Part model, mm, in its own coordinate system. Round coordinates to 2 decimals unless told otherwise and drop trailing zeros. Loops run counter-clockwise (first coordinate to the right, second up) from the corner with the lowest first, then second, coordinate; pieces in that order, holes last. Notation, with made-up numbers: M 37.25,-10.5 L 55.25,-10.5 A28 cw 55.25,8.5 Z; hole C -4.75,-39 d9. An arc over 180 degrees is marked long. Put each result on its own line as item: value. Start each with the question number.
1) Slice it at A-A on x = -97. Give the cut face in (y, z), then the cut area to 3 significant figures.
2) Probe line 1 along X through (y, z) = (2.75, -69); line 2 along X through (y, z) = (2, -39.5); line 3 along X through (y, z) = (5, 8). List the from-to ranges inside material, lowest first.
3) Slice it at B-B on y = 5. State how many separate pieces and enclosed holes the cut face has, then the cut area to 3 significant figures.
4) Drop a flat-ended pin along its axis: pin 1 Ø2 at (x, z) = (-12, 25) entering from +Y. Give the stop position or say it passes through.
```python
from build123d import *

# Parameters (mm, degrees)
SKETCH_1_R      = 1.7
SKETCH_1_R_2    = 2.15
SKETCH_1_R_3    = 2.65
SKETCH_1_R_4    = 10
EXTRUDE_2_DEPTH = 6


with BuildPart() as part:
    # 草图1 → 凸台-拉伸2 (new body)
    with BuildSketch(Plane(origin=(0, 0, 0), x_dir=(1, 0, 0), z_dir=(0, 1, 0))):
        with BuildLine():
            ThreePointArc((-125, -42), (-122.071067812, -49.071067812), (-115, -52))
            Line((-115, -52), (115, -52))
            ThreePointArc((115, -52), (122.071067812, -49.071067812), (125, -42))
            Line((125, -42), (125, 129))
            ThreePointArc((125, 129), (122.071067812, 136.071067812), (115, 139))
            Line((115, 139), (54.15581278, 139))
            ThreePointArc((54.15581278, 139), (50.06955504, 138.127020198), (46.696741396, 135.660499537))
            ThreePointArc((46.696741396, 135.660499537), (38.879992551, 123.497665763), (35.221472878, 109.510124102))
            ThreePointArc((35.221472878, 109.510124102), (33.603401462, 106.295315162), (30.245528585, 105))
            Line((30.245528585, 105), (-30.245528585, 105))
            ThreePointArc((-30.245528585, 105), (-33.603401462, 106.295315162), (-35.221472878, 109.510124102))
            ThreePointArc((-35.221472878, 109.510124102), (-38.879992551, 123.497665763), (-46.696741396, 135.660499537))
            ThreePointArc((-46.696741396, 135.660499537), (-50.06955504, 138.127020198), (-54.15581278, 139))
            Line((-54.15581278, 139), (-115, 139))
            ThreePointArc((-115, 139), (-122.071067812, 136.071067812), (-125, 129))
            Line((-125, 129), (-125, -42))
        make_face()
        with Locations(Location((-120, -35, 0), (0, 0, 270))):
            Circle(SKETCH_1_R, mode=Mode.SUBTRACT)
        with Locations(Location((-52, -35, 0), (0, 0, 270))):
            Circle(SKETCH_1_R, mode=Mode.SUBTRACT)
        with Locations(Location((-35, -25, 0), (0, 0, 270))):
            Circle(SKETCH_1_R_2, mode=Mode.SUBTRACT)
        with Locations(Location((-24.5, -25, 0), (0, 0, 270))):
            Circle(SKETCH_1_R, mode=Mode.SUBTRACT)
        with Locations(Location((-12, -25, 0), (0, 0, 270))):
            Circle(SKETCH_1_R, mode=Mode.SUBTRACT)
        with Locations(Location((-54, -15, 0), (0, 0, 270))):
            Circle(SKETCH_1_R, mode=Mode.SUBTRACT)
        with Locations(Location((-30, -15, 0), (0, 0, 270))):
            Circle(SKETCH_1_R, mode=Mode.SUBTRACT)
        with BuildLine():
            ThreePointArc((-76, 45), (-72.464466094, 43.535533906), (-71, 40))
            Line((-71, 40), (-71, -40))
            ThreePointArc((-71, -40), (-72.464466094, -43.535533906), (-76, -45))
            Line((-76, -45), (-106, -45))
            ThreePointArc((-106, -45), (-109.535533906, -43.535533906), (-111, -40))
            Line((-111, -40), (-111, 40))
            ThreePointArc((-111, 40), (-109.535533906, 43.535533906), (-106, 45))
            Line((-106, 45), (-76, 45))
        make_face(mode=Mode.SUBTRACT)
        with Locations(Location((-54, 15, 0), (0, 0, 270))):
            Circle(SKETCH_1_R, mode=Mode.SUBTRACT)
        with Locations(Location((-30, 15, 0), (0, 0, 270))):
            Circle(SKETCH_1_R, mode=Mode.SUBTRACT)
        with Locations(Location((-18.5, 30, 0), (0, 0, 270))):
            Circle(SKETCH_1_R, mode=Mode.SUBTRACT)
        with Locations(Location((12, -25, 0), (0, 0, 270))):
            Circle(SKETCH_1_R, mode=Mode.SUBTRACT)
        with Locations(Location((24.5, -25, 0), (0, 0, 270))):
            Circle(SKETCH_1_R, mode=Mode.SUBTRACT)
        with Locations(Location((35, -25, 0), (0, 0, 270))):
            Circle(SKETCH_1_R_2, mode=Mode.SUBTRACT)
        with Locations(Location((30, -15, 0), (0, 0, 270))):
            Circle(SKETCH_1_R, mode=Mode.SUBTRACT)
        with Locations(Location((54, -15, 0), (0, 0, 270))):
            Circle(SKETCH_1_R, mode=Mode.SUBTRACT)
        with Locations(Location((64, -31, 0), (0, 0, 270))):
            Circle(SKETCH_1_R, mode=Mode.SUBTRACT)
        with Locations(Location((118, -31, 0), (0, 0, 270))):
            Circle(SKETCH_1_R, mode=Mode.SUBTRACT)
        with BuildLine():
            add(Edge.make_bspline(
                [(-17, 10), (-17, -10.784609691), (8.5, -0.392304845), (34, 10), (8.5, 20.392304845), (-17, 30.784609691), (-17, 10)],
                knots=[0, 0, 0, 2.094395102, 2.094395102, 4.188790205, 4.188790205, 6.283185307, 6.283185307, 6.283185307], degree=2, weights=[1, 0.5, 1, 0.5, 1, 0.5, 1]))
        make_face(mode=Mode.SUBTRACT)
        with Locations(Location((30, 15, 0), (0, 0, 270))):
            Circle(SKETCH_1_R, mode=Mode.SUBTRACT)
        with Locations(Location((54, 15, 0), (0, 0, 270))):
            Circle(SKETCH_1_R, mode=Mode.SUBTRACT)
        with Locations(Location((18.5, 30, 0), (0, 0, 270))):
            Circle(SKETCH_1_R, mode=Mode.SUBTRACT)
        with BuildLine():
            ThreePointArc((76, -45), (72.464466094, -43.535533906), (71, -40))
            Line((71, -40), (71, 40))
            ThreePointArc((71, 40), (72.464466094, 43.535533906), (76, 45))
            Line((76, 45), (106, 45))
            ThreePointArc((106, 45), (109.535533906, 43.535533906), (111, 40))
            Line((111, 40), (111, -40))
            ThreePointArc((111, -40), (109.535533906, -43.535533906), (106, -45))
            Line((106, -45), (76, -45))
        make_face(mode=Mode.SUBTRACT)
        with Locations(Location((64, 31, 0), (0, 0, 270))):
            Circle(SKETCH_1_R, mode=Mode.SUBTRACT)
        with Locations(Location((118, 31, 0), (0, 0, 270))):
            Circle(SKETCH_1_R, mode=Mode.SUBTRACT)
        with Locations(Location((-120, 45, 0), (0, 0, 270))):
            Circle(SKETCH_1_R, mode=Mode.SUBTRACT)
        with BuildLine():
            ThreePointArc((-118, 75), (-115, 78), (-112, 75))
            Line((-112, 75), (-112, 60))
            ThreePointArc((-112, 60), (-115, 57), (-118, 60))
            Line((-118, 60), (-118, 75))
        make_face(mode=Mode.SUBTRACT)
        with Locations(Location((-52, 45, 0), (0, 0, 270))):
            Circle(SKETCH_1_R, mode=Mode.SUBTRACT)
        with BuildLine():
            ThreePointArc((-63, 51), (-66, 54), (-63, 57))
            Line((-63, 57), (-50, 57))
            ThreePointArc((-50, 57), (-47, 54), (-50, 51))
            Line((-50, 51), (-63, 51))
        make_face(mode=Mode.SUBTRACT)
        with Locations(Location((-35, 45, 0), (0, 0, 270))):
            Circle(SKETCH_1_R_2, mode=Mode.SUBTRACT)
        with BuildLine():
            ThreePointArc((-32, 60), (-35, 57), (-38, 60))
            Line((-38, 60), (-38, 75))
            ThreePointArc((-38, 75), (-35, 78), (-32, 75))
            Line((-32, 75), (-32, 60))
        make_face(mode=Mode.SUBTRACT)
        with Locations(Location((-18.5, 67, 0), (0, 0, 270))):
            Circle(SKETCH_1_R, mode=Mode.SUBTRACT)
        with Locations(Location((-24.5, 75, 0), (0, 0, 270))):
            Circle(SKETCH_1_R, mode=Mode.SUBTRACT)
        with BuildLine():
            ThreePointArc((-10.3, 75), (-12, 73.3), (-13.7, 75))
            ThreePointArc((-13.7, 75), (-12, 76.7), (-10.3, 75))
        make_face(mode=Mode.SUBTRACT)
        with Locations(Location((-115.149234169, 121.275702051, 0), (0, 0, 270))):
            Circle(SKETCH_1_R_3, mode=Mode.SUBTRACT)
        with Locations(Location((-90, 131, 0), (0, 0, 270))):
            Circle(SKETCH_1_R_3, mode=Mode.SUBTRACT)
        with Locations(Location((-60, 131, 0), (0, 0, 270))):
            Circle(SKETCH_1_R_3, mode=Mode.SUBTRACT)
        with Locations(Location((-90, 107, 0), (0, 0, 270))):
            Circle(SKETCH_1_R_2, mode=Mode.SUBTRACT)
        with BuildLine():
            ThreePointArc((-50, 121.5), (-47.5, 119), (-50, 116.5))
            Line((-50, 116.5), (-63, 116.5))
            ThreePointArc((-63, 116.5), (-65.5, 119), (-63, 121.5))
            Line((-63, 121.5), (-50, 121.5))
        make_face(mode=Mode.SUBTRACT)
        with Locations(Location((-60, 107, 0), (0, 0, 270))):
            Circle(SKETCH_1_R_2, mode=Mode.SUBTRACT)
        with Locations(Location((0, 48.5, 0), (0, 0, 270))):
            Circle(SKETCH_1_R_4, mode=Mode.SUBTRACT)
        with Locations(Location((35, 45, 0), (0, 0, 270))):
            Circle(SKETCH_1_R_2, mode=Mode.SUBTRACT)
        with BuildLine():
            ThreePointArc((50, 51), (47, 54), (50, 57))
            Line((50, 57), (63, 57))
            ThreePointArc((63, 57), (66, 54), (63, 51))
            Line((63, 51), (50, 51))
        make_face(mode=Mode.SUBTRACT)
        with Locations(Location((12, 75, 0), (0, 0, 270))):
            Circle(SKETCH_1_R, mode=Mode.SUBTRACT)
        with Locations(Location((18.5, 67, 0), (0, 0, 270))):
            Circle(SKETCH_1_R, mode=Mode.SUBTRACT)
        with Locations(Location((24.5, 75, 0), (0, 0, 270))):
            Circle(SKETCH_1_R, mode=Mode.SUBTRACT)
        with BuildLine():
            Line((38, 75), (38, 60))
            ThreePointArc((38, 60), (35, 57), (32, 60))
            Line((32, 60), (32, 75))
            ThreePointArc((32, 75), (35, 78), (38, 75))
        make_face(mode=Mode.SUBTRACT)
        with BuildLine():
            Line((118, 75), (118, 60))
            ThreePointArc((118, 60), (115, 57), (112, 60))
            Line((112, 60), (112, 75))
            ThreePointArc((112, 75), (115, 78), (118, 75))
        make_face(mode=Mode.SUBTRACT)
        with BuildLine():
            ThreePointArc((63, 122), (66, 119), (63, 116))
            Line((63, 116), (50, 116))
            ThreePointArc((50, 116), (47, 119), (50, 122))
            Line((50, 122), (63, 122))
        make_face(mode=Mode.SUBTRACT)
        with Locations(Location((60, 107, 0), (0, 0, 270))):
            Circle(SKETCH_1_R_2, mode=Mode.SUBTRACT)
        with Locations(Location((90, 107, 0), (0, 0, 270))):
            Circle(SKETCH_1_R_2, mode=Mode.SUBTRACT)
        with Locations(Location((60, 131, 0), (0, 0, 270))):
            Circle(SKETCH_1_R_3, mode=Mode.SUBTRACT)
        with Locations(Location((115.149234169, 121.275702051, 0), (0, 0, 270))):
            Circle(SKETCH_1_R_3, mode=Mode.SUBTRACT)
        with Locations(Location((90, 131, 0), (0, 0, 270))):
            Circle(SKETCH_1_R_3, mode=Mode.SUBTRACT)
    extrude(amount=EXTRUDE_2_DEPTH)


solid = part.part
```
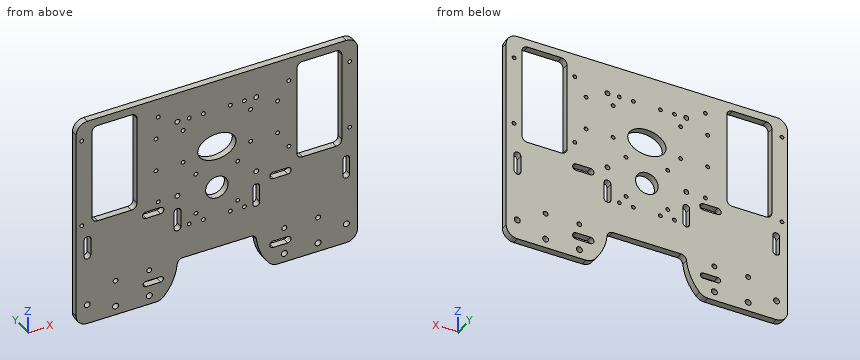
Recorded:
1. outline: M 0,-139 L 6,-139 L 6,-45 L 0,-45 Z; M 0,45 L 6,45 L 6,52 L 0,52 Z
1. area: 606 mm2
2. line 1: x = -125 to -118, -112 to -38, -32 to 32, 38 to 112, 118 to 125
2. line 2: x = -125 to -111, -71 to -4.36, 4.36 to 71, 111 to 125
2. line 3: x = -125 to -111, -71 to 71, 111 to 125
3. separate pieces: 1
3. enclosed holes: 54
3. area: 35,500 mm2
4. pin 1: passes through
